Input: part model. Units: mm. Frame: model coordinates. Face numbers are marked on the shaded views. A direction names the side the tool comes from. Give positions to 0.01 mm unless a question says otherwise; leave off trailing zeros. Order: outer loops, then holes, each group sorted by start corner. A loop starts at its lowest first (then second) coordinate and runs counter-clockwise, first axis right, second up. Notation, with made-up numbers: (66.5, 84.5) - (75.5, 84.5) arc R8 ccw to (75.5, 88.5) - close; hole circle Ø4 at (73, -16.5). An arc over 180 degrees is marked (long way). Use a Markdown table: item, result.
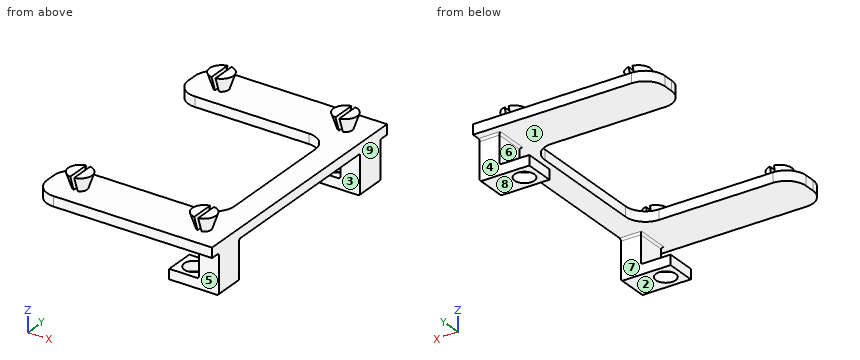
from build123d import *

# Parameters (mm, degrees)
IZIM1_W                     = 25
IZIM1_H                     = 26
Y_KSEKLIK_EKSTR_ZYON1_DEPTH = 1
IZIM12_W                    = 0.4
IZIM12_H                    = 1.5
KES_EKSTR_ZYON2_DEPTH       = 12
KES_EKSTR_ZYON2_DEPTH_BACK  = 25.3
IZIM13_W                    = 20
IZIM13_H                    = 16
KES_EKSTR_ZYON4_DEPTH       = 5
KES_EKSTR_ZYON4_DEPTH_BACK  = 4
RADYUS1_R                   = 2
IZIM14_W                    = 7
IZIM14_H                    = 26
KES_EKSTR_ZYON5_DEPTH       = 3
KES_EKSTR_ZYON5_DEPTH_BACK  = 3
RADYUS2_R                   = 2
IZIM17_W                    = 4
IZIM17_H                    = 3
Y_KSEKLIK_EKSTR_ZYON2_DEPTH = 2
IZIM18_W                    = 4
IZIM18_H                    = 3
Y_KSEKLIK_EKSTR_ZYON3_DEPTH = 1
IZIM19_R                    = 1
KES_EKSTR_ZYON6_DEPTH       = 1
RADYUS3_R                   = 0.2
RADYUS3_OF_AYNALAMA2_R      = 0.2


with BuildPart() as part:
    # Çizim1 → Yükseklik-Ekstrüzyon1 (new body)
    with BuildSketch(Plane.XY):
        Rectangle(IZIM1_W, IZIM1_H)
    extrude(amount=Y_KSEKLIK_EKSTR_ZYON1_DEPTH)

    # Çizim9 → Döndür1 (revolve)
    with BuildSketch(Plane(origin=(0, 10.5, 0), x_dir=(1, 0, 0), z_dir=(0, 1, 0))):
        Polygon((-2.5, -1), (-2.5, -2.5), (-3.7, -2.5), (-3.2, -1), align=None)
    d_nd_r1 = revolve(axis=Axis((-2.5, 10.5, 1), (0, 0, 1)))

    # Çizim11 → Döndür2 (revolve)
    with BuildSketch(Plane(origin=(0, 10.5, 0), x_dir=(1, 0, 0), z_dir=(0, 1, 0))):
        Polygon((10, -1), (10, -2.5), (8.8, -2.5), (9.3, -1), align=None)
    d_nd_r2 = revolve(axis=Axis((10, 10.5, 1), (0, 0, 1)))

    # Aynalama1: Döndür1, Döndür2 across plane
    add(d_nd_r1.mirror(Plane.ZX))
    add(d_nd_r2.mirror(Plane.ZX))

    # Çizim12 → Kes-Ekstrüzyon2 (cut, two sides)
    with BuildSketch(Plane(origin=(0, 10.5, 0), x_dir=(1, 0, 0), z_dir=(0, 1, 0))) as kes_ekstr_zyon2_sk:
        with Locations((-2.5, -1.75)):
            Rectangle(IZIM12_W, IZIM12_H)
        with Locations((10, -1.75)):
            Rectangle(IZIM12_W, IZIM12_H)
    extrude(amount=KES_EKSTR_ZYON2_DEPTH, mode=Mode.SUBTRACT)
    extrude(kes_ekstr_zyon2_sk.sketch, amount=-KES_EKSTR_ZYON2_DEPTH_BACK, mode=Mode.SUBTRACT)

    # Çizim13 → Kes-Ekstrüzyon4 (cut, two sides)
    with BuildSketch(Plane.XY) as kes_ekstr_zyon4_sk:
        Rectangle(IZIM13_W, IZIM13_H)
    extrude(amount=KES_EKSTR_ZYON4_DEPTH, mode=Mode.SUBTRACT)
    extrude(kes_ekstr_zyon4_sk.sketch, amount=-KES_EKSTR_ZYON4_DEPTH_BACK, mode=Mode.SUBTRACT)

    # Radyus1
    radyus1_edges = [part.edges().sort_by_distance(p)[0] for p in [
        (10, 8, 0.5),
        (-10, 8, 0.5),
        (-10, -8, 0.5),
        (10, -8, 0.5),
    ]]
    fillet(radyus1_edges, radius=RADYUS1_R)

    # Çizim14 → Kes-Ekstrüzyon5 (cut, two sides)
    with BuildSketch(Plane.XY) as kes_ekstr_zyon5_sk:
        with Locations((-9, 0)):
            Rectangle(IZIM14_W, IZIM14_H)
    extrude(amount=KES_EKSTR_ZYON5_DEPTH, mode=Mode.SUBTRACT)
    extrude(kes_ekstr_zyon5_sk.sketch, amount=-KES_EKSTR_ZYON5_DEPTH_BACK, mode=Mode.SUBTRACT)

    # Radyus2
    radyus2_edges = [part.edges().sort_by_distance(p)[0] for p in [
        (-5.5, -8, 0.5),
        (-5.5, 13, 0.5),
        (-5.5, -13, 0.5),
        (-5.5, 8, 0.5),
    ]]
    fillet(radyus2_edges, radius=RADYUS2_R)

    # Çizim17 → Yükseklik-Ekstrüzyon2 (add)
    with BuildSketch(Plane(origin=(10.5, 0, 0), x_dir=(0, 0, -1), z_dir=(1, 0, 0))):
        with Locations((2, 10.5)):
            Rectangle(IZIM17_W, IZIM17_H)
    y_kseklik_ekstr_zyon2 = extrude(amount=Y_KSEKLIK_EKSTR_ZYON2_DEPTH)

    # Çizim18 → Yükseklik-Ekstrüzyon3 (add)
    with BuildSketch(Plane(origin=(0, 0, -4), x_dir=(-1, 0, 0), z_dir=(0, 0, -1))):
        with Locations((-9.5, 10.5)):
            Rectangle(IZIM18_W, IZIM18_H)
    y_kseklik_ekstr_zyon3 = extrude(amount=-Y_KSEKLIK_EKSTR_ZYON3_DEPTH)

    # Çizim19 → Kes-Ekstrüzyon6 (cut)
    with BuildSketch(Plane(origin=(0, 0, -4), x_dir=(-1, 0, 0), z_dir=(0, 0, -1))):
        with Locations((-9, 10.5)):
            Circle(IZIM19_R)
    kes_ekstr_zyon6 = extrude(amount=-KES_EKSTR_ZYON6_DEPTH, mode=Mode.SUBTRACT)

    # Radyus3
    radyus3_edges = [part.edges().sort_by_distance(p)[0] for p in [
        (10.5, 10.5, 0),
        (11.5, 12, 0),
        (11.5, 9, 0),
        (12.5, 10.5, -4),
        (10.5, 10.5, -3),
    ]]
    fillet(radyus3_edges, radius=RADYUS3_R)

    # Aynalama2: Yükseklik-Ekstrüzyon2, Yükseklik-Ekstrüzyon3, Kes-Ekstrüzyon6 across plane
    add(y_kseklik_ekstr_zyon2.mirror(Plane.ZX))
    add(y_kseklik_ekstr_zyon3.mirror(Plane.ZX))
    add(kes_ekstr_zyon6.mirror(Plane.ZX), mode=Mode.SUBTRACT)

    # Radyus3 of Aynalama2
    radyus3_of_aynalama2_edges = [part.edges().sort_by_distance(p)[0] for p in [
        (10.5, -10.5, 0),
        (11.5, -12, 0),
        (11.5, -9, 0),
        (12.5, -10.5, -4),
        (10.5, -10.5, -3),
    ]]
    fillet(radyus3_of_aynalama2_edges, radius=RADYUS3_OF_AYNALAMA2_R)


solid = part.part
1. Section query D-D (y = -2). Return loops of the section in (x, z).
Response:
| item | result |
|---|---|
| outline | (10, 0) - (12.5, 0) - (12.5, 1) - (10, 1) - close |
2. Section query A-A (x = 5). Return loops of the section in (y, z), then the cut area to 3 significant figures.
Response:
| item | result |
|---|---|
| outline | (-13, 0) - (-8, 0) - (-8, 1) - (-13, 1) - close; (8, 0) - (13, 0) - (13, 1) - (8, 1) - close |
| area | 10.0 mm^2 |
3. Pin query (flat end, axial travel): pin 1 (1.1 mm diameter, centred on x = 10.5, z = -3, fed in from -Y); pin 2 (0.5 mm diameter, centred on y = 10.5, z = -3.5, fed in from -X); pin 3 (1.5 mm diameter, centred on y = -10, z = -1, fed in from -X); pin 4 (3 mm diameter, centred on x = -3, z = 1.5, fed in from +Y). Return the tip coordinate at first contact, or that it passes through.
Response:
| item | result |
|---|---|
| pin 1 | stops at y = -12 |
| pin 2 | stops at x = 7.5 |
| pin 3 | stops at x = 10.5 |
| pin 4 | stops at y = 13 |
4. Section query C-C (z = -2). Return loops of the section in (x, y), then the cut area to 3 significant figures.
Response:
| item | result |
|---|---|
| outline | (10.5, -12) - (12.5, -12) - (12.5, -9) - (10.5, -9) - close; (10.5, 9) - (12.5, 9) - (12.5, 12) - (10.5, 12) - close |
| area | 12.0 mm^2 |
5. Set-up query: the marked faces 5, 6, 7, 8 and 9. Return all of +Z, -Z, +X, -X, +Y, -Y with unobstructed straight access to the full face (end or side cutting, diameter ignored); none if empty.
Response:
| item | result |
|---|---|
| face 5 | -Z, +X, -X, -Y |
| face 6 | -X, +Y, -Y |
| face 7 | -Z, +X, -X |
| face 8 | -Z, +X, -X, +Y, -Y |
| face 9 | +Z, -Z, +X, +Y, -Y |
6. Mould query, pull axis Y, two halves, no side actions, for the marked faces 1, 2, 3 and 4. Classes: pulls with the +Y half, pulls with the -Y half, needs draft (parallel to the pull), parting line crosses it, or undercut.
Response:
| item | result |
|---|---|
| face 1 | undercut |
| face 2 | needs draft |
| face 3 | undercut |
| face 4 | pulls with the +Y half |
7. Material intervals for line 1 along Y through (x, z) = (9, -3.25); line 2 along Y through (x, z) = (11.75, -1); line 3 along X through (y, z) = (-10.5, -3.25), sorted ascending.
Response:
| item | result |
|---|---|
| line 1 | y = -12 to -11.5, -9.5 to -9, 9 to 9.5, 11.5 to 12 |
| line 2 | y = -12 to -9, 9 to 12 |
| line 3 | x = 7.5 to 8, 10 to 12.5 |
